Geometry check sheet. Reference: the model listing, model coordinates, mm. A direction names the side the tool comes from. Coordinates: 2 decimals unless noted, no trailing zeros. Write each loop counter-clockwise with the first axis right and the second up, starting at its lowest first coordinate (ties: lowest second). Pieces come first, ordered by that corner, then holes. Notation, with made-up numbers: (-39, 5.25) -> (-7, 5.25) arc R15 ccw to (-7, 22.25) -> close; hole circle Ø6 at (75.5, 38.25). An arc over 180 degrees is marked (long way). Answer in a Markdown table with one row per item. Add a question column.
1. Depth check by flat-ended pin: P1, Ø2.5, axis at x = 5, z = 5, coming from the -Y side; P2, Ø3.5, axis at x = 1, y = 16.5, coming from the -Z side; P3, Ø5.5, axis at x = 0, y = 40, coming from the -Z side. Enter the tip coordinate at first touch or a pass-through.
2. Cross-section at A-A on y = 40. Record the cut outline in (x, z) (3 decimals), and give its area (3 significant figures).
3. Set-up check for faces 4 (the flat face through (6.479, -22, -1)), 5 (the flat face through (2.815, 40, 15)), 6 (the flat face through (0, 1, 6.7)), 7 (the flat face through (13.8, 42.65, -3.06)), 8 (the cylindrical face through (-18, 39, 0)): record each of +Z, -Z, +X, -X, +Y, -Y from which the full face is reachable in a straight line by a thin tool's end or side.
4. Cross-section at C-C on y = 5.5. Record the cut outline in (x, z).
5. Cross-section at B-B on y = 23. Record the cut outline in (x, z), and give its area (3 significant figures).
6. Cross-section at D-D on z = 0. Give the number of separate pieces and of enclosed holes in the cut face, and give its area (3 significant figures).
7. Mould release check, pull along X, two halves, no side actions. Record for faces 1 (the flat face through (1, 14, 14.4)), 2 (the cylindrical face through (-8.29, 31.33, 0.24)), 3 (the flat face through (2.815, 30, 15)): pulls with the +X half, pulls with the -X half, needs draft (parallel to the pull), parting line crosses it, or undercut.
8. Scan lines: L1, parallel to Y at x = 0, z = -8.75; L2, parallel to Z at x = 0, y = 0.8; L3, parallel to Y at x = 3, z = -10. Record each from-to range of solid material in increasing order. Write a range as from..to.
```python
from build123d import *
from build123d.topology import SkipClean

# Parameters (mm, degrees)
SKETCH_1_R          = 18
EXTRUDE_1_DEPTH     = 45
SKETCH_2_R          = 19.5
EXTRUDE_2_DEPTH     = 2
SKETCH_3_W          = 10.25
SKETCH_3_H          = 10.25
CUT_EXTRUDE_1_DEPTH = 40
EXTRUDE_3_DEPTH     = 15
SKETCH1_R           = 18
BOSS_EXTRUDE1_DEPTH = 20
SKETCH3_R           = 18
BOSS_EXTRUDE2_DEPTH = 7
SKETCH4_W           = 10.2
SKETCH4_H           = 10.2
CUT_EXTRUDE2_DEPTH  = 27
CUT_EXTRUDE4_DEPTH  = 25
BOSS_EXTRUDE3_DEPTH = 3
SKETCH9_W           = 36
SKETCH9_H           = 22
CUT_EXTRUDE5_DEPTH  = 8
SKETCH10_R          = 3.7
SKETCH10_W          = 3
SKETCH10_H          = 2
CUT_EXTRUDE6_DEPTH  = 10
SKETCH11_R          = 2
CUT_EXTRUDE7_DEPTH  = 102
SKETCH15_R          = 18
CUT_EXTRUDE9_DEPTH  = 27
CUT_EXTRUDE11_DEPTH = 20
SKETCH18_R          = 1.5
CUT_EXTRUDE12_DEPTH = 63.62188116
SKETCH19_R          = 3
CUT_EXTRUDE13_DEPTH = 3
BOSS_EXTRUDE5_DEPTH = 22
CUT_EXTRUDE16_DEPTH = 4
CUT_EXTRUDE17_DEPTH = 6
CUT_EXTRUDE18_DEPTH = 63.62188116
FILLET2_R           = 5
SKETCH30_W          = 18.8
SKETCH30_H          = 10
CUT_EXTRUDE20_DEPTH = 3
CHAMFER1_SIZE       = 1
CHAMFER1_SIZE2      = 2.747477419
CHAMFER2_SIZE       = 1
CHAMFER2_SIZE2      = 2.747477419
SKETCH37_W          = 9
SKETCH37_H          = 9
SKETCH37_R          = 2
BOSS_EXTRUDE7_DEPTH = 15
CUT_EXTRUDE22_DEPTH = 15
CUT_EXTRUDE23_REACH = 69.856
SKETCH40_W          = 4.363156696
SKETCH40_H          = 4.363156696
CUT_EXTRUDE24_DEPTH = 10
FILLET7_R           = 6


with BuildPart() as part:
    # Эскиз1 → Бобышка-Вытянуть1 (new body)
    with BuildSketch(Plane(origin=(0, 0, 0), x_dir=(1, 0, 0), z_dir=(0, 1, 0))):
        with Locations(Location((0, 0, 0), (0, 0, 90))):
            Circle(SKETCH_1_R)
    extrude(amount=EXTRUDE_1_DEPTH)

    # Эскиз2 → Бобышка-Вытянуть2 (add)
    with BuildSketch(Plane(origin=(0, 45, 0), x_dir=(1, 0, 0), z_dir=(0, 1, 0))):
        with Locations(Location((0, 0, 0), (0, 0, 270))):
            Circle(SKETCH_2_R)
    extrude(amount=EXTRUDE_2_DEPTH)

    # Эскиз3 → Вырез-Вытянуть1 (cut)
    with BuildSketch(Plane(origin=(0, 47, 0), x_dir=(1, 0, 0), z_dir=(0, 1, 0))):
        Rectangle(SKETCH_3_W, SKETCH_3_H)
    extrude(amount=-CUT_EXTRUDE_1_DEPTH, mode=Mode.SUBTRACT)

    # Эскиз4 → Бобышка-Вытянуть3 (add)
    with BuildSketch(Plane.XZ):
        with BuildLine():
            Line((5.142300877, -6.128355545), (11.570176974, -13.788799976))
            ThreePointArc((11.570176974, -13.788799976), (17.937391115, -1.5), (13.69961987, 11.675633406))
            Line((13.69961987, 11.675633406), (5.142300877, 4.38257561))
            Line((5.142300877, 4.38257561), (5.142300877, -6.128355545))
        make_face()
    extrude(amount=EXTRUDE_3_DEPTH)

    # Sketch1 → Boss-Extrude1 (add)
    with BuildSketch(Plane.XZ.offset(15)):
        with Locations(Location((0, 0, 0), (0, 0, 270))):
            Circle(SKETCH1_R)
    extrude(amount=BOSS_EXTRUDE1_DEPTH)

    # Sketch3 → Boss-Extrude2 (add)
    with BuildSketch(Plane.XZ.offset(35)):
        with Locations(Location((0, 0, 0), (0, 0, 270))):
            Circle(SKETCH3_R)
    extrude(amount=BOSS_EXTRUDE2_DEPTH)

    # Sketch4 → Cut-Extrude2 (cut)
    with BuildSketch(Plane.XZ.offset(42)):
        Rectangle(SKETCH4_W, SKETCH4_H)
    extrude(amount=-CUT_EXTRUDE2_DEPTH, mode=Mode.SUBTRACT)

    # Sketch6 → Cut-Extrude4 (cut)
    with BuildSketch(Plane.XZ):
        with BuildLine():
            Line((0, 18), (0, -18))
            ThreePointArc((0, -18), (-18, 0), (0, 18))
        make_face()
    extrude(amount=-CUT_EXTRUDE4_DEPTH, mode=Mode.SUBTRACT)

    # Sketch8 → Boss-Extrude3 (add)
    with BuildSketch(Plane.XZ):
        with BuildLine():
            Line((0, -18), (0, 18))
            ThreePointArc((0, 18), (-18, 0), (0, -18))
        make_face()
    extrude(amount=-BOSS_EXTRUDE3_DEPTH)

    # Sketch9 → Cut-Extrude5 (cut)
    with BuildSketch(Plane.ZY):
        with Locations((0, 14)):
            Rectangle(SKETCH9_W, SKETCH9_H)
    extrude(amount=-CUT_EXTRUDE5_DEPTH, mode=Mode.SUBTRACT)

    # Sketch10 → Cut-Extrude6 (cut)
    with BuildSketch(Plane.XZ):
        with Locations(Location((0, 0, 0), (0, 0, 270))):
            Circle(SKETCH10_R)
        with Locations((0, 7.7)):
            Rectangle(SKETCH10_W, SKETCH10_H)
    extrude(amount=-CUT_EXTRUDE6_DEPTH, mode=Mode.SUBTRACT)

    # Sketch11 → Cut-Extrude7 (cut)
    with BuildSketch(Plane.XZ.offset(42)):
        with Locations(Location((12, 0, 0), (0, 0, 270))):
            Circle(SKETCH11_R)
    extrude(amount=-CUT_EXTRUDE7_DEPTH, mode=Mode.SUBTRACT)

    # Sketch15 → Cut-Extrude9 (cut)
    with BuildSketch(Plane.XZ.offset(42)):
        with Locations(Location((0, 0, 0), (0, 0, 310))):
            Circle(SKETCH15_R)
    extrude(amount=-CUT_EXTRUDE9_DEPTH, mode=Mode.SUBTRACT)

    # Sketch17 → Cut-Extrude11 (cut)
    with BuildSketch(Plane.XZ.offset(-25)):
        with BuildLine():
            Line((5.916079783, -17), (-5.916079783, -17))
            ThreePointArc((-5.916079783, -17), (0, -18), (5.916079783, -17))
        make_face()
        with BuildLine():
            Line((5.916079783, 17), (-5.916079783, 17))
            ThreePointArc((-5.916079783, 17), (0, 18), (5.916079783, 17))
        make_face()
    extrude(amount=-CUT_EXTRUDE11_DEPTH, mode=Mode.SUBTRACT)

    # Sketch18 → Cut-Extrude12 (cut, through all)
    with BuildSketch(Plane.XY.offset(-17)):
        with Locations(Location((0, 30, 0), (0, 0, 180))):
            Circle(SKETCH18_R)
        with Locations(Location((0, 40, 0), (0, 0, 180))):
            Circle(SKETCH18_R)
    extrude(amount=CUT_EXTRUDE12_DEPTH, mode=Mode.SUBTRACT)

    # Sketch19 → Cut-Extrude13 (cut)
    with BuildSketch(Plane.XY.offset(-17)):
        with Locations((0, 30)):
            Circle(SKETCH19_R)
        with Locations((0, 40)):
            Circle(SKETCH19_R)
    extrude(amount=CUT_EXTRUDE13_DEPTH, mode=Mode.SUBTRACT)

    # Sketch23 → Boss-Extrude5 (add)
    with SkipClean():  # the faces are left unmerged after this step: merging them gives an invalid solid
        with BuildSketch(Plane(origin=(0, 3, 0), x_dir=(1, 0, 0), z_dir=(0, 1, 0))):
            with BuildLine():
                Line((0, -14.4), (8, -14.4))
                Line((8, -14.4), (8, -16.124515497))
                ThreePointArc((8, -16.124515497), (4.108449894, -17.524857759), (0, -18))
                Line((0, -18), (0, -14.4))
            make_face()
            with BuildLine():
                Line((0, 14.4), (8, 14.4))
                Line((8, 14.4), (8, 16.124515497))
                ThreePointArc((8, 16.124515497), (4.108449894, 17.524857759), (0, 18))
                Line((0, 18), (0, 14.4))
            make_face()
        extrude(amount=BOSS_EXTRUDE5_DEPTH)

    # Sketch25 → Cut-Extrude16 (cut)
    with SkipClean():  # the faces are left unmerged after this step: merging them gives an invalid solid
        with BuildSketch(Plane.XY.offset(17)):
            Polygon((-2.814582562, 28.375), (0, 26.75), (2.814582562, 28.375), (2.814582562, 31.625), (0, 33.25), (-2.814582562, 31.625), align=None)
            Polygon((-2.814582562, 41.625), (-2.814582562, 38.375), (0, 36.75), (2.814582562, 38.375), (2.814582562, 41.625), (0, 43.25), align=None)
        extrude(amount=-CUT_EXTRUDE16_DEPTH, mode=Mode.SUBTRACT)

    # Sketch26 → Cut-Extrude17 (cut)
    with SkipClean():  # the faces are left unmerged after this step: merging them gives an invalid solid
        with BuildSketch(Plane(origin=(0, 47, 0), x_dir=(1, 0, 0), z_dir=(0, 1, 0))):
            Polygon((8.449295844, -2.05), (12, -4.1), (15.550704156, -2.05), (15.550704156, 2.05), (12, 4.1), (8.449295844, 2.05), align=None)
        extrude(amount=-CUT_EXTRUDE17_DEPTH, mode=Mode.SUBTRACT)

    # Sketch27 → Cut-Extrude18 (cut, through all)
    with SkipClean():  # the faces are left unmerged after this step: merging them gives an invalid solid
        with BuildSketch(Plane.XY.offset(17)):
            with BuildLine():
                Line((-20, 36.547005384), (-20, 25))
                Line((-20, 25), (0, 25))
                ThreePointArc((0, 25), (-9.324199199, 31.944024015), (-20, 36.547005384))
            make_face()
        extrude(amount=-CUT_EXTRUDE18_DEPTH, mode=Mode.SUBTRACT)

    # Fillet2
    fillet2_edges = [part.edges().sort_by_distance(p)[0] for p in [
        (8, 14, -14.4),
        (8, 14, 14.4),
    ]]
    fillet(fillet2_edges, radius=FILLET2_R)

    # Sketch30 → Cut-Extrude20 (cut)
    with SkipClean():  # the faces are left unmerged after this step: merging them gives an invalid solid
        with BuildSketch(Plane.ZY.offset(-8)):
            with Locations((0, 8)):
                Rectangle(SKETCH30_W, SKETCH30_H)
        extrude(amount=-CUT_EXTRUDE20_DEPTH, mode=Mode.SUBTRACT)

    # Chamfer1
    chamfer1_edges = [part.edges().sort_by_distance(p)[0] for p in [
        (5.125, 47, 0),
        (0, 47, -5.125),
        (-5.125, 47, 0),
        (0, 47, 5.125),
    ]]
    chamfer1_side = [part.faces().sort_by_distance(p)[0] for p in [
        (0, 47, -18.948456711),
    ]]
    chamfer(chamfer1_edges, length=CHAMFER1_SIZE, length2=CHAMFER1_SIZE2, reference=chamfer1_side[0])

    # Chamfer2
    chamfer2_edges = [part.edges().sort_by_distance(p)[0] for p in [
        (8.449295844, 47, 0),
        (10.224647922, 47, 3.075),
        (13.775352078, 47, 3.075),
        (15.550704156, 47, 0),
        (13.775352078, 47, -3.075),
        (10.224647922, 47, -3.075),
    ]]
    chamfer2_side = [part.faces().sort_by_distance(p)[0] for p in [
        (6.676543289, 47, 0),
    ]]
    chamfer(chamfer2_edges, length=CHAMFER2_SIZE, length2=CHAMFER2_SIZE2, reference=chamfer2_side[0])

    # Sketch37 → Boss-Extrude7 (add)
    with SkipClean():  # the faces are left unmerged after this step: merging them gives an invalid solid
        with BuildSketch(Plane.XZ.offset(15)):
            with Locations((10.978822628, -0.872889968)):
                Rectangle(SKETCH37_W, SKETCH37_H)
            with Locations(Location((12, 0, 0), (0, 0, 270))):
                Circle(SKETCH37_R, mode=Mode.SUBTRACT)
        extrude(amount=BOSS_EXTRUDE7_DEPTH)

    # Sketch38 → Cut-Extrude22 (cut)
    with SkipClean():  # the faces are left unmerged after this step: merging them gives an invalid solid
        with BuildSketch(Plane.XZ.offset(15)):
            with BuildLine():
                Line((5.142300877, -6.128355545), (5.142300877, 4.38257561))
                ThreePointArc((5.142300877, 4.38257561), (5.978822628, -0.872889968), (5.142300877, -6.128355545))
            make_face()
        extrude(amount=-CUT_EXTRUDE22_DEPTH, mode=Mode.SUBTRACT)

    # Cut-Extrude23: up to this face of the body (flat: up to its plane)
    cut_extrude23_end = Plane(part.part.faces().sort_by_distance((9.450359937, 13, 0))[0])
    # Sketch39 → Cut-Extrude23 (cut, up to the picked face)
    with BuildSketch(Plane.XZ.offset(15), mode=Mode.PRIVATE) as cut_extrude23_sk1:
        with BuildLine():
            Line((7.420733648, -7.372889968), (15.420733648, -7.372889968))
            ThreePointArc((15.420733648, -7.372889968), (13.728515389, -10.030415688), (11.598853111, -12.352178848))
            Line((11.598853111, -12.352178848), (7.420733648, -7.372889968))
        make_face()
    cut_extrude23_tool1 = split(extrude(cut_extrude23_sk1.sketch, amount=-CUT_EXTRUDE23_REACH, mode=Mode.PRIVATE), bisect_by=cut_extrude23_end, keep=Keep.BOTH, mode=Mode.PRIVATE)
    add(cut_extrude23_tool1.solids().sort_by(Axis((11.596211, -15, -9.081847), (0, 1, 0)))[0], mode=Mode.SUBTRACT)

    # Sketch40 → Cut-Extrude24 (cut)
    with SkipClean():  # the faces are left unmerged after this step: merging them gives an invalid solid
        with BuildSketch(Plane(origin=(0, 3, 0), x_dir=(1, 0, 0), z_dir=(0, 1, 0))):
            with Locations((9.602311996, 9.554468316)):
                Rectangle(SKETCH40_W, SKETCH40_H)
        extrude(amount=CUT_EXTRUDE24_DEPTH, mode=Mode.SUBTRACT)

    # Fillet7
    fillet7_edges = [part.edges().sort_by_distance(p)[0] for p in [
        (5.142300877, -7.5, 4.38257561),
        (5.142300877, -7.5, -6.128355545),
    ]]
    fillet(fillet7_edges, radius=FILLET7_R)


solid = part.part
```
Results found:
| question | item | result |
|---|---|---|
| 1 | P1 | stops at y = 0 |
| 1 | P2 | stops at z = -18 |
| 1 | P3 | stops at z = -14 |
| 2 | outline | (-5.916, -17) -> (-3, -17) -> (-3, -14) -> (-1.5, -14) -> (-1.5, -5.125) -> (-5.125, -5.125) -> (-5.125, 5.125) -> (-1.5, 5.125) -> (-1.5, 13) -> (-2.815, 13) -> (-2.815, 17) -> (-5.916, 17) arc R18 ccw to start; (1.5, -14) -> (3, -14) -> (3, -17) -> (5.916, -17) arc R18 ccw to (5.916, 17) -> (2.815, 17) -> (2.815, 13) -> (1.5, 13) -> (1.5, 5.125) -> (5.125, 5.125) -> (5.125, -5.125) -> (1.5, -5.125) -> close; hole circle Ø4 at (12, 0) |
| 2 | area | 794 mm^2 |
| 3 | face 4 | +Z, -Z, -X, -Y |
| 3 | face 5 | +Z |
| 3 | face 6 | -Y |
| 3 | face 7 | +Y |
| 3 | face 8 | -X, -Y |
| 4 | outline | (0, -18) arc R18 ccw to (0, 18) -> (0, 14.4) -> (3, 14.4) arc R5 cw to (8, 9.4) -> (11, 9.4) -> (11, 1.73) arc R2 cw (long way) to (11, -1.73) -> (11, -7.37) -> (15.42, -7.37) arc R18 cw to (11.6, -12.35) -> (11.08, -11.74) -> (7.42, -11.74) arc R5 cw to (3, -14.4) -> (0, -14.4) -> close |
| 5 | outline | (0, -18) arc R18 ccw to (0, 18) -> (0, 14.4) -> (3, 14.4) arc R5 cw to (8, 9.4) -> (8, -9.4) arc R5 cw to (3, -14.4) -> (0, -14.4) -> close; hole circle Ø4 at (12, 0) |
| 5 | area | 277 mm^2 |
| 6 | separate pieces | 5 |
| 6 | enclosed holes | 0 |
| 6 | area | 739 mm^2 |
| 7 | face 1 | needs draft |
| 7 | face 2 | pulls with the -X half |
| 7 | face 3 | undercut |
| 8 | L1 | y = 0..3, 25..28.5, 31.5..38.5, 41.5..47 |
| 8 | L2 | z = -18..-3.7, 3.7..6.7, 8.7..18 |
| 8 | L3 | y = 0..3, 25..47 |
